Geometry check sheet. Reference: the model listing, model coordinates, mm. Face numbers are marked on the shaded views. Round coordinates to 2 decimals unless told otherwise and drop trailing zeros. Order: outer loops, then holes, each group sorted by start corner. A loop starts at its lowest first (then second) coordinate and runs counter-clockwise, first axis right, second up. Notation, with made-up numbers: (17.25, 78) -> (21.25, 78) arc R25 cw to (21.25, 92) -> close; hole circle Ø1 at (18.5, 50). An arc over 180 degrees is marked (long way). Use a Markdown table: item, result. Add a question column.
Item 1: Sectioned sample at C-C, the plane z = 0.1. Record the cut outline in (x, y) (3 decimals).
Item 2: Sectioned sample at A-A, the plane y = 0. Record the cut outline in (x, z) (3 decimals), and give its area (3 significant figures).
Item 3: Sectioned sample at D-D, the plane y = -1.5. Record the cut outline in (x, z).
Item 4: Material ranges on probe 1 along Y at (x, z) = (0, 0.3); probe 2 along Z at (x, y) = (-3, 0.75); probe 3 along Y at (x, z) = (2.25, 0.35), recorded low to high. Write a range as [from, to].
Item 5: Gauge pin test, flat end, axial feed: pin 1 Ø2 at (x, y) = (2, -1.5) entering from +Z. Record the tip position at first contact, or that the pin passes through.
Item 6: Mould release check, pull along X, two halves, no side actions. Record for the marked faces 1, 2 and 3: pulls with the +X half, pulls with the -X half, needs draft (parallel to the pull), parting line crosses it, or undercut.
Item 7: Sectioned sample at B-B, the plane x = 0. Record the cut outline in (y, z), and give its area (3 significant figures).
from build123d import *

# Parameters (mm, degrees)
SKETCH_1_R      = 3.9
SKETCH_1_R_2    = 0.5
EXTRUDE_1_DEPTH = 0.8
SKETCH_2_W      = 2.5
SKETCH_2_H      = 1.5
EXTRUDE_2_DEPTH = 0.1


with BuildPart() as part:
    # 草图1 → 凸台-拉伸1 (new body)
    with BuildSketch(Plane.XY):
        Circle(SKETCH_1_R)
        Circle(SKETCH_1_R_2, mode=Mode.SUBTRACT)
        with BuildLine():
            Line((-2.405, 0.8), (-2.395, 0.8))
            ThreePointArc((-2.395, 0.8), (-2.133370491, 0.691629509), (-2.025, 0.43))
            Line((-2.025, 0.43), (-2.025, -0.43))
            ThreePointArc((-2.025, -0.43), (-2.133370491, -0.691629509), (-2.395, -0.8))
            Line((-2.395, -0.8), (-2.405, -0.8))
            ThreePointArc((-2.405, -0.8), (-2.666629509, -0.691629509), (-2.775, -0.43))
            Line((-2.775, -0.43), (-2.775, 0.43))
            ThreePointArc((-2.775, 0.43), (-2.666629509, 0.691629509), (-2.405, 0.8))
        make_face(mode=Mode.SUBTRACT)
        with BuildLine():
            Line((2.395, 0.8), (2.405, 0.8))
            ThreePointArc((2.405, 0.8), (2.666629509, 0.691629509), (2.775, 0.43))
            Line((2.775, 0.43), (2.775, -0.43))
            ThreePointArc((2.775, -0.43), (2.666629509, -0.691629509), (2.405, -0.8))
            Line((2.405, -0.8), (2.395, -0.8))
            ThreePointArc((2.395, -0.8), (2.133370491, -0.691629509), (2.025, -0.43))
            Line((2.025, -0.43), (2.025, 0.43))
            ThreePointArc((2.025, 0.43), (2.133370491, 0.691629509), (2.395, 0.8))
        make_face(mode=Mode.SUBTRACT)
    extrude(amount=EXTRUDE_1_DEPTH)

    # 草图2 → 凸台-拉伸2 (add)
    with BuildSketch(Plane.XY.offset(0.8)):
        with Locations((0, 2)):
            Rectangle(SKETCH_2_W, SKETCH_2_H)
        with Locations((0, -2)):
            Rectangle(SKETCH_2_W, SKETCH_2_H)
    extrude(amount=EXTRUDE_2_DEPTH)


solid = part.part
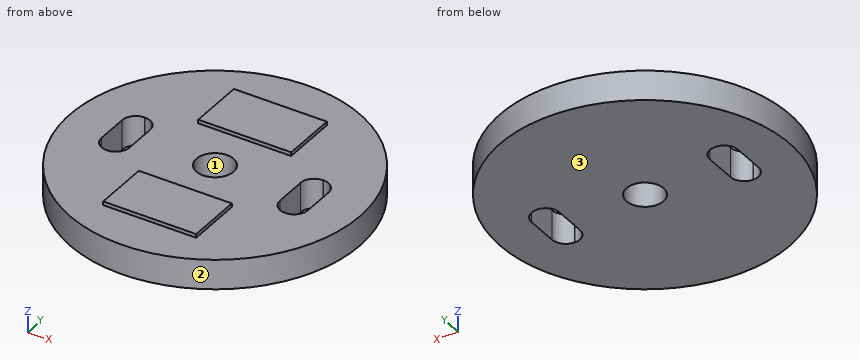
Found:
| question | item | result |
|---|---|---|
| 1 | outline | circle Ø7.8 at (0, 0); hole (-2.775, -0.43) arc R0.37 ccw to (-2.405, -0.8) -> (-2.395, -0.8) arc R0.37 ccw to (-2.025, -0.43) -> (-2.025, 0.43) arc R0.37 ccw to (-2.395, 0.8) -> (-2.405, 0.8) arc R0.37 ccw to (-2.775, 0.43) -> close; hole circle Ø1 at (0, 0); hole (2.025, -0.43) arc R0.37 ccw to (2.395, -0.8) -> (2.405, -0.8) arc R0.37 ccw to (2.775, -0.43) -> (2.775, 0.43) arc R0.37 ccw to (2.405, 0.8) -> (2.395, 0.8) arc R0.37 ccw to (2.025, 0.43) -> close |
| 2 | outline | (-3.9, 0) -> (-2.775, 0) -> (-2.775, 0.8) -> (-3.9, 0.8) -> close; (-2.025, 0) -> (-0.5, 0) -> (-0.5, 0.8) -> (-2.025, 0.8) -> close; (0.5, 0) -> (2.025, 0) -> (2.025, 0.8) -> (0.5, 0.8) -> close; (2.775, 0) -> (3.9, 0) -> (3.9, 0.8) -> (2.775, 0.8) -> close |
| 2 | area | 4.24 mm2 |
| 3 | outline | (-3.6, 0) -> (3.6, 0) -> (3.6, 0.8) -> (1.25, 0.8) -> (1.25, 0.9) -> (-1.25, 0.9) -> (-1.25, 0.8) -> (-3.6, 0.8) -> close |
| 4 | probe 1 | y = [-3.9, -0.5], [0.5, 3.9] |
| 4 | probe 2 | z = [0, 0.8] |
| 4 | probe 3 | y = [-3.19, -0.77], [0.77, 3.19] |
| 5 | pin 1 | stops at z = 0.9 |
| 6 | face 1 | undercut |
| 6 | face 2 | parting line crosses it |
| 6 | face 3 | needs draft |
| 7 | outline | (-3.9, 0) -> (-0.5, 0) -> (-0.5, 0.8) -> (-1.25, 0.8) -> (-1.25, 0.9) -> (-2.75, 0.9) -> (-2.75, 0.8) -> (-3.9, 0.8) -> close; (0.5, 0) -> (3.9, 0) -> (3.9, 0.8) -> (2.75, 0.8) -> (2.75, 0.9) -> (1.25, 0.9) -> (1.25, 0.8) -> (0.5, 0.8) -> close |
| 7 | area | 5.74 mm2 |
